Source: CAD feature listing. Evaluate the final solid. Frame: model axes, mm. Round coordinates to 2 decimals unless told otherwise and drop trailing zeros. Write each loop counter-clockwise with the first axis right and the second up, starting at its lowest first coordinate (ties: lowest second). Pieces come first, ordered by that corner, then holes. Notation, with made-up numbers: M 84,25 L 137,25 A27 ccw 137,62 Z; hole C 37.5,3.25 d1. An arc over 180 degrees is marked long. Answer in a Markdown table with one row per item. Add a question column.
Item 1: Cut plane D-D on x = 17. Return loops of the section in (y, z), and give its area (3 significant figures).
Item 2: Material intervals for probe 1 along Y at (x, z) = (6, -3.25); probe 2 along Z at (x, y) = (-4, -52.5); probe 3 along X at (y, z) = (-60, -2.25), sorted ascending.
Item 3: Cut plane B-B on z = -1.75. Return loops of the section in (x, y), and give its area (3 significant figures).
Item 4: Contact query for flat-ended pins moving along their axis: pin 1 (6.5 mm diameter, centred on x = 5.31, y = -61.62, fed in from +Z); pin 2 (19.5 mm diameter, centred on x = 9, y = -42, fed in from -Z); pin 3 (1 mm diameter, centred on x = 6.5, z = -2, fed in from -Y). Output: stop coordinate, or through.
Item 5: Cut plane A-A on x = -1.5. Return loops of the section in (y, z).
Item 6: Cut plane C-C on y = -44. Return loops of the section in (x, z), and give its area (3 significant figures).
from build123d import *

# Parameters (mm, degrees)
SKETCH1_R             = 8
SKETCH1_R_2           = 2
BOSS_EXTRUDE1_DEPTH   = 3.5
BOSS_EXTRUDE1_2_DEPTH = 3.5
BOSS_EXTRUDE1_3_DEPTH = 3.5
SKETCH4_W             = 60
SKETCH4_H             = 6.5
EXTRUDE_THIN1_DEPTH   = 3.5
FILLET1_R             = 3
SKETCH_1_R            = 8
SKETCH_1_R_2          = 2
EXTRUDE_1_DEPTH       = 3
FILLET_2_R            = 3


with BuildPart() as part:
    # Sketch1 → Boss-Extrude1 (new body)
    with BuildSketch(Plane.XY):
        with Locations((-29.621497739, -38.307799929)):
            Circle(SKETCH1_R)
        with Locations((-29.621497739, -38.307799929)):
            Circle(SKETCH1_R_2, mode=Mode.SUBTRACT)
    extrude(amount=-BOSS_EXTRUDE1_DEPTH)



with BuildPart() as body_2:
    # Sketch1 → Boss-Extrude1 2 (new body)
    with BuildSketch(Plane.XY):
        with Locations((40.247017363, -38.307799929)):
            Circle(SKETCH1_R)
        with Locations((40.247017363, -38.307799929)):
            Circle(SKETCH1_R_2, mode=Mode.SUBTRACT)
    extrude(amount=-BOSS_EXTRUDE1_2_DEPTH)


with BuildPart() as body_3:
    # Sketch1 → Boss-Extrude1 3 (new body)
    with BuildSketch(Plane.XY):
        with Locations((5.312759812, -61.622980593)):
            Circle(SKETCH1_R)
        with Locations((5.312759812, -61.622980593)):
            Circle(SKETCH1_R_2, mode=Mode.SUBTRACT)
    extrude(amount=-BOSS_EXTRUDE1_3_DEPTH)


with BuildPart() as part_1:
    add(part.part)

    add(body_2.part)  # Extrude-Thin1 merges body 2

    add(body_3.part)  # Extrude-Thin1 merges body 3
    # Sketch4 → Extrude-Thin1 (add)
    with BuildSketch(Plane.XY):
        with Locations((5.312759812, -38.307799929)):
            Rectangle(SKETCH4_W, SKETCH4_H)
        Polygon((-26.435040402, -44.341786144), (-1.481999294, -60.995486618), (2.126302475, -55.588994378), (-22.826738632, -38.935293904), align=None)
        Polygon((12.107518918, -60.995486618), (37.060560026, -44.341786144), (33.452258256, -38.935293904), (8.499217149, -55.588994378), align=None)
    extrude(amount=-EXTRUDE_THIN1_DEPTH)

    # Fillet1
    fillet1_edges = [part_1.edges().sort_by_distance(p)[0] for p in [
        (-18.897311611, -41.557799929, -1.75),
        (1.036606698, -54.861729633, -1.75),
        (9.588912926, -54.861729633, -1.75),
        (29.522831235, -41.557799929, -1.75),
    ]]
    fillet(fillet1_edges, radius=FILLET1_R)

    # 草图1 → 凸台-拉伸1 (add)
    with BuildSketch(Plane(origin=(0, 0, -3.5), x_dir=(-1, 0, 0), z_dir=(0, 0, -1))):
        with Locations(Location((29.621497739, -38.307799929, 0), (0, 0, 156.030517682))):
            Circle(SKETCH_1_R)
        with Locations(Location((29.621497739, -38.307799929, 0), (0, 0, 180))):
            Circle(SKETCH_1_R_2, mode=Mode.SUBTRACT)
    extrude(amount=EXTRUDE_1_DEPTH)

    # 圆角2
    # the kernel refuses this fillet: 3 mm, written as the material it adds along each edge
    with BuildSketch(Plane(origin=(-22.31140198, -35.057799929, -3.5), x_dir=(1, 0, 0), z_dir=(0, 0, 1)), Plane(origin=(-2.571695072, -60.268221873, -3.5), x_dir=(-0.8317680369208076, 0.5551233491368437, 0), z_dir=(0, 0, 1)), Plane(origin=(35.970864249, -45.069050889, -3.5), x_dir=(-0.8317680369208071, -0.5551233491368445, 0), z_dir=(0, 0, 1))) as fillet_2_piece_1:
        with BuildLine():
            CenterArc((1.741837737, 3), FILLET_2_R, 214.623535479, 55.376464521)
            ThreePointArc((-0.726871399, 1.295454545), (-0.333303043, 0.664634517), (0, 0))
            Line((0, 0), (1.741837737, 0))
        make_face()
    extrude(amount=3.5)
    with BuildSketch(Plane(origin=(32.936921604, -35.057799929, -3.5), x_dir=(0.4893293145989847, 0.8720990894812859, 0), z_dir=(0, 0, 1)), Plane(origin=(-25.345344625, -45.069050889, -3.5), x_dir=(-0.8911310507438419, -0.45374601970725476, 0), z_dir=(0, 0, 1))) as fillet_2_piece_2:
        with BuildLine():
            CenterArc((1.763965003, 2.987043048), FILLET_2_R, 209.296508898, 55.376464521)
            Line((-0.852332266, 1.519055104), (0, 0))
            ThreePointArc((0, 0), (0.742722106, 0.034551872), (1.485444213, 0))
        make_face()
    extrude(amount=3.5)
    with BuildSketch(Plane(origin=(13.197214696, -60.268221873, -3.5), x_dir=(0.8317680369208036, 0.5551233491368496, 0), z_dir=(0, 0, 1))) as fillet_2_piece_3:
        with BuildLine():
            CenterArc((1.741837737, -3), FILLET_2_R, 90, 55.376464521)
            ThreePointArc((-0.726871399, -1.295454545), (-0.333303043, -0.664634517), (0, 0))
            Line((0, 0), (1.741837737, 0))
        make_face()
    extrude(amount=3.5)


solid = part_1.part
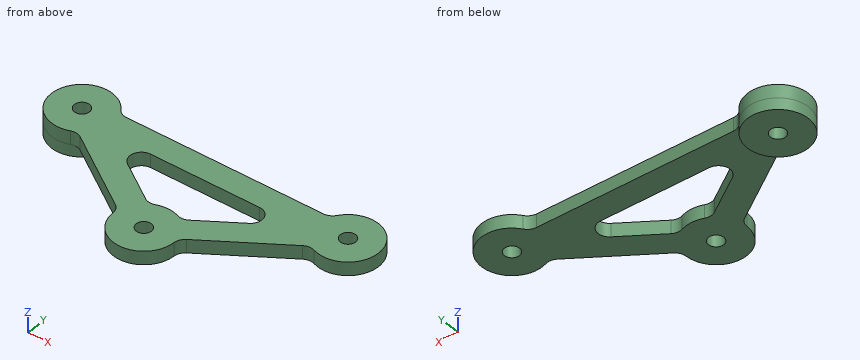
Results below:
| question | item | result |
|---|---|---|
| 1 | outline | M -57.73,-3.5 L -49.92,-3.5 L -49.92,0 L -57.73,0 Z; M -41.56,-3.5 L -35.06,-3.5 L -35.06,0 L -41.56,0 Z |
| 1 | area | 50.1 mm2 |
| 2 | probe 1 | -69.59 to -63.5, -59.74 to -53.65, -41.56 to -35.06 |
| 2 | probe 2 | -3.5 to 0 |
| 2 | probe 3 | -3.28 to 4.14, 6.48 to 13.91 |
| 3 | outline | M -26.67,-45.74 A3 cw -23.9,-46.04 L -4.02,-59.3 A3 cw -2.69,-61.75 A8 ccw 13.31,-61.75 A3 cw 14.65,-59.3 L 34.52,-46.04 A3 cw 37.29,-45.74 A8 ccw long 33.66,-33.76 A3 cw 31.2,-35.06 L -20.57,-35.06 A3 cw -23.04,-33.76 A8 ccw long Z; hole C -29.62,-38.31 d4; hole M -10.66,-47.05 L -0.41,-53.89 A3 ccw 2.36,-54.19 A8 cw 8.27,-54.19 A3 ccw 11.04,-53.89 L 21.29,-47.05 A3 ccw 19.62,-41.56 L -9,-41.56 A3 ccw Z; hole C 5.31,-61.62 d4; hole C 40.25,-38.31 d4 |
| 3 | area | 1,300 mm2 |
| 4 | pin 1 | z = 0 |
| 4 | pin 2 | z = -3.5 |
| 4 | pin 3 | y = -69.59 |
| 5 | outline | M -65.82,-3.5 L -53.17,-3.5 L -53.17,0 L -65.82,0 Z; M -41.56,-3.5 L -35.06,-3.5 L -35.06,0 L -41.56,0 Z |
| 6 | outline | M -35.24,-6.5 L -24,-6.5 L -24,-3.5 L -11.95,-3.5 L -11.95,0 L -35.24,0 Z; M 22.57,-3.5 L 45.87,-3.5 L 45.87,0 L 22.57,0 Z |
| 6 | area | 197 mm2 |
